from build123d import *

# Parameters (mm, degrees)
SKETCH1_W           = 60
SKETCH1_H           = 60
SKETCH1_R           = 2.5
SKETCH1_R_2         = 22
SKETCH1_R_3         = 18.5
BOSS_EXTRUDE1_DEPTH = 5
BOSS_EXTRUDE2_START = 5
SKETCH1_3_R         = 22
SKETCH1_3_R_2       = 18.5
BOSS_EXTRUDE2_DEPTH = 20
FILLET1_R           = 2
BOSS_EXTRUDE6_DEPTH = 25
SKETCH5_R           = 2
BOSS_EXTRUDE7_DEPTH = 2


with BuildPart() as part:
    # Sketch1 → Boss-Extrude1 (new body)
    with BuildSketch(Plane(origin=(0, 0, 0), x_dir=(1, 0, 0), z_dir=(0, 1, 0))):
        Rectangle(SKETCH1_W, SKETCH1_H)
        with Locations(Location((22.778174593, 22.778174593, 0), (0, 0, 270))):
            Circle(SKETCH1_R, mode=Mode.SUBTRACT)
        with Locations(Location((22.778174593, -22.778174593, 0), (0, 0, 270))):
            Circle(SKETCH1_R, mode=Mode.SUBTRACT)
        with Locations(Location((-22.778174593, -22.778174593, 0), (0, 0, 270))):
            Circle(SKETCH1_R, mode=Mode.SUBTRACT)
        Circle(SKETCH1_R_2, mode=Mode.SUBTRACT)
        with Locations(Location((-22.778174593, 22.778174593, 0), (0, 0, 270))):
            Circle(SKETCH1_R, mode=Mode.SUBTRACT)
        Circle(SKETCH1_R_2)
        Circle(SKETCH1_R_3, mode=Mode.SUBTRACT)
        Circle(SKETCH1_R_3)
    extrude(amount=BOSS_EXTRUDE1_DEPTH)

    # Sketch1<3> → Boss-Extrude2 (add)
    with BuildSketch(Plane(origin=(0, 0, 0), x_dir=(1, 0, 0), z_dir=(0, 1, 0)).offset(BOSS_EXTRUDE2_START)):
        with Locations(Location((0, 0, 0), (0, 0, 270))):
            Circle(SKETCH1_3_R)
        Circle(SKETCH1_3_R_2, mode=Mode.SUBTRACT)
        Circle(SKETCH1_3_R_2)
    extrude(amount=BOSS_EXTRUDE2_DEPTH)

    # Sketch3 → Cut-Revolve4 (revolve, cut)
    with BuildSketch(Plane.XY):
        with BuildLine():
            Line((0, 16.001538563), (0, 25))
            Line((0, 25), (-18.5, 25))
            ThreePointArc((-18.5, 25), (-17.906501611, 20.351645447), (-16.164086481, 16.001538563))
            Line((-16.164086481, 16.001538563), (0, 16.001538563))
        make_face()
        with BuildLine():
            Line((0, 6.5), (0, 16.001538563))
            Line((0, 16.001538563), (-16.164086481, 16.001538563))
            ThreePointArc((-16.164086481, 16.001538563), (-9.374925691, 9.051308258), (0, 6.5))
        make_face()
    revolve(axis=Axis((0, 6.5, 0), (0, 1, 0)), mode=Mode.SUBTRACT)

    # Fillet1
    fillet1_edges = [part.edges().sort_by_distance(p)[0] for p in [
        (-30, 2.5, 30),
        (-30, 2.5, -30),
        (30, 2.5, -30),
        (30, 2.5, 30),
    ]]
    fillet(fillet1_edges, radius=FILLET1_R)

    # Sketch4 → Boss-Extrude6 (add)
    with BuildSketch(Plane(origin=(0, 5, 0), x_dir=(1, 0, 0), z_dir=(0, 1, 0))):
        with BuildLine():
            ThreePointArc((3, 23.8117618), (0, 24), (-3, 23.8117618))
            Line((-3, 23.8117618), (-3, 21.794494718))
            ThreePointArc((-3, 21.794494718), (0, 22), (3, 21.794494718))
            Line((3, 21.794494718), (3, 23.8117618))
        make_face()
        with BuildLine():
            Line((-3, -21.794494718), (-3, -23.8117618))
            ThreePointArc((-3, -23.8117618), (0, -24), (3, -23.8117618))
            Line((3, -23.8117618), (3, -21.794494718))
            ThreePointArc((3, -21.794494718), (0, -22), (-3, -21.794494718))
        make_face()
    extrude(amount=BOSS_EXTRUDE6_DEPTH)

    # Sketch5 → Boss-Extrude7 (add)
    with BuildSketch(Plane(origin=(0, 25, 0), x_dir=(1, 0, 0), z_dir=(0, 1, 0))):
        with BuildLine():
            ThreePointArc((30, 2), (29.414213562, 3.414213562), (28, 4))
            Line((28, 4), (21.633307653, 4))
            ThreePointArc((21.633307653, 4), (22, 0), (21.633307653, -4))
            Line((21.633307653, -4), (28, -4))
            ThreePointArc((28, -4), (29.414213562, -3.414213562), (30, -2))
            Line((30, -2), (30, 2))
        make_face()
        with Locations(Location((27, 0, 0), (0, 0, 270))):
            Circle(SKETCH5_R, mode=Mode.SUBTRACT)
        with BuildLine():
            ThreePointArc((-21.633307653, -4), (-22, 0), (-21.633307653, 4))
            Line((-21.633307653, 4), (-28, 4))
            ThreePointArc((-28, 4), (-29.414213562, 3.414213562), (-30, 2))
            Line((-30, 2), (-30, -2))
            ThreePointArc((-30, -2), (-29.414213562, -3.414213562), (-28, -4))
            Line((-28, -4), (-21.633307653, -4))
        make_face()
        with Locations(Location((-27, 0, 0), (0, 0, 270))):
            Circle(SKETCH5_R, mode=Mode.SUBTRACT)
    extrude(amount=-BOSS_EXTRUDE7_DEPTH)


solid = part.part
Could you check a few things on this model? Use its own coordinates, in mm. A direction names the side the tool comes from. Round coordinates to 2 decimals unless told otherwise and drop trailing zeros. Order: outer loops, then holes, each group sorted by start corner. A loop starts at its lowest first (then second) coordinate and runs counter-clockwise, first axis right, second up. Notation, with made-up numbers: M 55,-15.75 L 103,-15.75 A24 cw 103,-0.75 Z; hole C 87,31 d1. An arc over 180 degrees is marked long. One line per item, written item: value.
(1) Imagine slicing it at A-A (z = 0). Write out the boundary of the cut face in (x, y).
Ans:
outline: M -30,0 L 30,0 L 30,5 L 22,5 L 22,23 L 25,23 L 25,25 L 18.5,25 A18.5 cw -18.5,25 L -25,25 L -25,23 L -22,23 L -22,5 L -30,5 Z; M -30,23 L -29,23 L -29,25 L -30,25 Z; M 29,23 L 30,23 L 30,25 L 29,25 Z
(2) If we mould it in two halves opening along Y, with no side actions, what happens to faces 6 (the flat face through (24.8, 23, -0.1)), 7 (the flat face through (0, 2, -30))? For each: released by +Y, released by -Y, zero draft, split by the parting line, or undercut.
Ans:
face 6: undercut
face 7: zero draft
(3) Imagine slicing it at D-D (y = 4). Write out the boundary of the cut face in (x, z), and give its area (3 significant figures).
Ans:
outline: M -30,-28 A2 ccw -28,-30 L 28,-30 A2 ccw 30,-28 L 30,28 A2 ccw 28,30 L -28,30 A2 ccw -30,28 Z; hole C -22.78,-22.78 d5; hole C -22.78,22.78 d5; hole C 22.78,-22.78 d5; hole C 22.78,22.78 d5
area: 3,520 mm^2
(4) Imagine slicing it at C-C (x = 27). Write out the boundary of the cut face in (y, z), and give its area (3 significant figures).
Ans:
outline: M 0,-30 L 5,-30 L 5,30 L 0,30 Z; M 23,-4 L 25,-4 L 25,-2 L 23,-2 Z; M 23,2 L 25,2 L 25,4 L 23,4 Z
area: 308 mm^2
(5) I'm going to push flat-ended pins straight in: P1, Ø1.6, axis at y = 15.5, z = -23.5, coming from the -X side; P2, Ø4, axis at x = -22, y = 12.5, coming from the +Z side; P3, Ø12, axis at x = -2, y = 11.5, coming from the -Z side. Where does each tip first touch, or does it pass through?
Ans:
P1: stops at x = -3
P2: stops at z = 9.17
P3: stops at z = -24
(6) Which directions (+Z, -Z, +X, -X, +Y, -Y) give clear straight access to the entire face, cutting with the end or side of a thin tool? Please do faces 1 (the cylindrical face through (0, 17, 24)), 2 (the cylindrical face through (29.4, 24.01, 3.43)), 3 (the cylindrical face through (-29.43, 24.01, 3.4)), 4 (the flat face through (-25, 24, -4)), 5 (the cylindrical face through (-29, 24, 0)).
Ans:
face 1: +Z, +Y
face 2: +Z, +X, +Y
face 3: +Z, -X, +Y
face 4: -Z, -X, +Y
face 5: +Y
(7) Imagine slicing it at B-B (y = 28). Write out the boundary of the cut face in (x, z), and give its area (3 significant figures).
Ans:
outline: M -3,-23.81 A24 ccw 3,-23.81 L 3,-21.79 A22 cw -3,-21.79 Z; M -3,21.79 A22 cw 3,21.79 L 3,23.81 A24 ccw -3,23.81 Z
area: 24.1 mm^2
(8) I need wall thicknesses on line 1 along X through (y, z) = (24.1, 0); line 2 along X through (y, z) = (2, 22); line 3 along Y through (x, z) = (-5, -23). Which ranges of each line are inside material? Lowest first, please. Write a range as from..to.
Ans:
line 1: x = -30..-29, -25..-18.48, 18.48..25, 29..30
line 2: x = -30..-25.15, -20.4..20.4, 25.15..30
line 3: y = 0..5
